```python
from build123d import *

# Parameters (mm, degrees)
BOSS_EXTRUDE1_DEPTH = 1.9685
SKETCH2_R           = 0.4064
CUT_EXTRUDE1_DEPTH  = 24.55446458
SKETCH3_R           = 2.0828
CUT_EXTRUDE2_DEPTH  = 0.2286
SKETCH4_R           = 0.9525
CUT_EXTRUDE3_DEPTH  = 24.536462381
BOSS_EXTRUDE2_START = 1.2446
SKETCH5_R           = 3.00355
SKETCH5_R_2         = 1.73355
BOSS_EXTRUDE2_DEPTH = 1.2446


with BuildPart() as part:
    # Sketch1 → Boss-Extrude1 (new body)
    with BuildSketch(Plane.XY):
        with BuildLine():
            Line((2.020348077, -2.2225), (-2.020348077, -2.2225))
            ThreePointArc((-2.020348077, -2.2225), (0, -3.00355), (2.020348077, -2.2225))
        make_face()
        with BuildLine():
            Line((2.020348077, 2.2225), (-2.020348077, 2.2225))
            ThreePointArc((-2.020348077, 2.2225), (-3.00355, 0), (-2.020348077, -2.2225))
            Line((-2.020348077, -2.2225), (2.020348077, -2.2225))
            ThreePointArc((2.020348077, -2.2225), (2.746773477, -1.215132942), (3.00355, 0))
            ThreePointArc((3.00355, 0), (2.746773477, 1.215132942), (2.020348077, 2.2225))
        make_face()
        with BuildLine():
            ThreePointArc((2.020348077, 2.2225), (0, 3.00355), (-2.020348077, 2.2225))
            Line((-2.020348077, 2.2225), (2.020348077, 2.2225))
        make_face()
        with BuildLine():
            Line((21.8821, 2.2225), (2.020348077, 2.2225))
            ThreePointArc((2.020348077, 2.2225), (2.746773477, 1.215132942), (3.00355, 0))
            ThreePointArc((3.00355, 0), (2.746773477, -1.215132942), (2.020348077, -2.2225))
            Line((2.020348077, -2.2225), (21.8821, -2.2225))
            ThreePointArc((21.8821, -2.2225), (22.900844734, -1.31254669), (23.2791, 0))
            ThreePointArc((23.2791, 0), (22.900844734, 1.31254669), (21.8821, 2.2225))
        make_face()
        with BuildLine():
            Line((-2.020348077, 2.2225), (-21.8821, 2.2225))
            ThreePointArc((-21.8821, 2.2225), (-22.900844734, 1.31254669), (-23.2791, 0))
            ThreePointArc((-23.2791, 0), (-22.900844734, -1.31254669), (-21.8821, -2.2225))
            Line((-21.8821, -2.2225), (-2.020348077, -2.2225))
            ThreePointArc((-2.020348077, -2.2225), (-3.00355, 0), (-2.020348077, 2.2225))
        make_face()
    extrude(amount=BOSS_EXTRUDE1_DEPTH)

    # Sketch2 → Cut-Extrude1 (cut, through all)
    with BuildSketch(Plane.XY.offset(1.9685)):
        with Locations((-20.7391, 0)):
            Circle(SKETCH2_R)
        with Locations((-18.1737, 0)):
            Circle(SKETCH2_R)
        with Locations((-15.6083, 0)):
            Circle(SKETCH2_R)
        with Locations((-13.0429, 0)):
            Circle(SKETCH2_R)
        with Locations((-10.4775, 0)):
            Circle(SKETCH2_R)
        with Locations((-7.9121, 0)):
            Circle(SKETCH2_R)
        with Locations((-5.3467, 0)):
            Circle(SKETCH2_R)
        with Locations(Location((5.3467, 0, 0), (0, 0, 180))):
            Circle(SKETCH2_R)
        with Locations(Location((7.9121, 0, 0), (0, 0, 180))):
            Circle(SKETCH2_R)
        with Locations(Location((10.4775, 0, 0), (0, 0, 180))):
            Circle(SKETCH2_R)
        with Locations(Location((13.0429, 0, 0), (0, 0, 180))):
            Circle(SKETCH2_R)
        with Locations(Location((15.6083, 0, 0), (0, 0, 180))):
            Circle(SKETCH2_R)
        with Locations(Location((18.1737, 0, 0), (0, 0, 180))):
            Circle(SKETCH2_R)
        with Locations(Location((20.7391, 0, 0), (0, 0, 180))):
            Circle(SKETCH2_R)
    extrude(amount=-CUT_EXTRUDE1_DEPTH, mode=Mode.SUBTRACT)

    # Sketch3 → Cut-Extrude2 (cut)
    with BuildSketch(Plane.XY.offset(1.9685)):
        Circle(SKETCH3_R)
    extrude(amount=-CUT_EXTRUDE2_DEPTH, mode=Mode.SUBTRACT)

    # Sketch4 → Cut-Extrude3 (cut, through all)
    with BuildSketch(Plane.XY.offset(1.7399)):
        Circle(SKETCH4_R)
    extrude(amount=-CUT_EXTRUDE3_DEPTH, mode=Mode.SUBTRACT)

    # Sketch5 → Boss-Extrude2 (add)
    with BuildSketch(Plane(origin=(0, 0, 0), x_dir=(-1, 0, 0), z_dir=(0, 0, -1)).offset(BOSS_EXTRUDE2_START)):
        Circle(SKETCH5_R)
        Circle(SKETCH5_R_2, mode=Mode.SUBTRACT)
    extrude(amount=-BOSS_EXTRUDE2_DEPTH)


solid = part.part
```
Can you work these out from the model? Positions are in its coordinate system, mm. A direction names the side the tool comes from. Coordinates: 2 decimals unless noted, no trailing zeros. Order: outer loops, then holes, each group sorted by start corner. A loop starts at its lowest first (then second) coordinate and runs counter-clockwise, first axis right, second up. Notation, with made-up numbers: (76, -18) - (89, -18) arc R29 cw to (89, 19) - close; hole circle Ø1 at (82, -18.5). An arc over 180 degrees is marked (long way). Answer in a Markdown table with one row per item.
1. For faces 4 (the flat face through (1, -1, 0)), 5 (the cylindrical face through (-0.21, -0.93, 0.88)), 6 (the flat face through (12, 2.222, 1)), which set-ups out of +Z, -Z, +X, -X, +Y, -Y let a thin tool reach every point of the face, with its end or its side?
Reply:
| item | result |
|---|---|
| face 4 | -Z |
| face 5 | +Z, -Z |
| face 6 | +Z, -Z, +X, +Y |
2. If I drill on line 1 along Y through (x, z) = (8, 1.45); line 2 along Y through (x, z) = (0, -0.25); line 3 along Z through (x, y) = (18.5, -1.5), over which ranges is the centre line in solid material (lowest first)?
Reply:
| item | result |
|---|---|
| line 1 | y = -2.22 to -0.4, 0.4 to 2.22 |
| line 2 | y = -3 to -1.73, 1.73 to 3 |
| line 3 | z = 0 to 1.97 |
3. Suppose I cut it at B-B (z = -0.6). Please give me the cut outline in (x, y), and give its area (3 significant figures).
Reply:
| item | result |
|---|---|
| outline | circle Ø6.01 at (0, 0); hole circle Ø3.47 at (0, 0) |
| area | 18.9 mm^2 |
4. Suppose I cut it at A-A (x = 0). Please give me the cut outline in (y, z).
Reply:
| item | result |
|---|---|
| outline | (-3, -1.24) - (-1.73, -1.24) - (-1.73, 0) - (-0.95, 0) - (-0.95, 1.74) - (-2.08, 1.74) - (-2.08, 1.97) - (-3, 1.97) - close; (0.95, 0) - (1.73, 0) - (1.73, -1.24) - (3, -1.24) - (3, 1.97) - (2.08, 1.97) - (2.08, 1.74) - (0.95, 1.74) - close |
5. For pin 1 (1 mm diameter, centred on x = -11, z = 1.5, fed in from +Y); pin 2 (2 mm diameter, centred on x = -12.5, y = 1, fed in from -Z); pin 3 (2 mm diameter, centred on x = 0, y = 0, fed in from +Z); pin 4 (1.2 mm diameter, centred on x = 0, y = 0, fed in from +Z), each with a flat end and sliding along its axis, tell me the tip position at first contact or that it passes through.
Reply:
| item | result |
|---|---|
| pin 1 | stops at y = 2.22 |
| pin 2 | stops at z = 0 |
| pin 3 | stops at z = 1.74 |
| pin 4 | passes through |
6. If we mould it in two halves opening along Y, with no side actions, what happens to faces 1 (the flat face through (-0.3, -2.6, 1.968)), 2 (the flat face through (-12, 2.222, 1)), 3 (the cylindrical face through (-16.014, 0.018, 0.998))? For each: pulls with the +Y half, pulls with the -Y half, needs draft (parallel to the pull), parting line crosses it, or undercut.
Reply:
| item | result |
|---|---|
| face 1 | needs draft |
| face 2 | pulls with the +Y half |
| face 3 | undercut |
